Could you check a few things on this model? Use its own coordinates, in mm. A direction names the side the tool comes from. Give positions to 0.01 mm unless a question says otherwise; leave off trailing zeros. Loops run counter-clockwise (first coordinate to the right, second up) from the corner with the lowest first, then second, coordinate; pieces in that order, holes last. Notation, with made-up numbers: M 0,74 L 33,74 A18 ccw 33,99 Z; hole C 16.25,-30.75 d3. An arc over 180 degrees is marked long. Use CSV: the item, a comma, the result in double quotes.
```python
from build123d import *

# Parameters (mm, degrees)
PAD_DEPTH       = 4
SKETCH001_R     = 3.75
PAD001_DEPTH    = 9
SKETCH002_R     = 2.15
POCKET_DEPTH    = 7
CHAMFER_SIZE    = 1.5
CHAMFER001_SIZE = 1.5
CHAMFER002_SIZE = 1.5
FILLET_R        = 5
FILLET001_R     = 5


with BuildPart() as part:
    # Sketch → Pad (new body)
    with BuildSketch(Plane.XY):
        Polygon((0, 0), (20, 0), (30, 10), (30, 20), (20, 30), (0, 30), align=None)
        with BuildLine():
            ThreePointArc((4.5, 6.5), (3, 5), (4.5, 3.5))
            Line((4.5, 3.5), (7, 3.5))
            ThreePointArc((7, 3.5), (8.5, 5), (7, 6.5))
            Line((7, 6.5), (4.5, 6.5))
        make_face(mode=Mode.SUBTRACT)
        with BuildLine():
            ThreePointArc((4.5, 26.5), (3, 25), (4.5, 23.5))
            Line((4.5, 23.5), (7, 23.5))
            ThreePointArc((7, 23.5), (8.5, 25), (7, 26.5))
            Line((7, 26.5), (4.5, 26.5))
        make_face(mode=Mode.SUBTRACT)
        with BuildLine():
            ThreePointArc((23.5, 16.5), (22, 15), (23.5, 13.5))
            Line((23.5, 13.5), (26, 13.5))
            ThreePointArc((26, 13.5), (27.5, 15), (26, 16.5))
            Line((26, 16.5), (23.5, 16.5))
        make_face(mode=Mode.SUBTRACT)
    extrude(amount=PAD_DEPTH)

    # Sketch001 → Pad001 (join)
    with BuildSketch(Plane.XY):
        with Locations((15, 25.5)):
            Circle(SKETCH001_R)
        with Locations((15, 4.5)):
            Circle(SKETCH001_R)
    extrude(amount=PAD001_DEPTH)

    # Sketch002 → Pocket (cut)
    with BuildSketch(Plane.XY.offset(9)):
        with Locations((15, 25.5)):
            Circle(SKETCH002_R)
        with Locations((15, 4.5)):
            Circle(SKETCH002_R)
    extrude(amount=-POCKET_DEPTH, mode=Mode.SUBTRACT)

    # Chamfer
    chamfer_edges = [part.edges().sort_by_distance(p)[0] for p in [
        (3, 5, 4),
        (5.75, 6.5, 4),
        (8.5, 5, 4),
        (5.75, 3.5, 4),
    ]]
    chamfer(chamfer_edges, length=CHAMFER_SIZE)

    # Chamfer001
    chamfer001_edges = [part.edges().sort_by_distance(p)[0] for p in [
        (3, 25, 4),
        (5.75, 26.5, 4),
        (8.5, 25, 4),
        (5.75, 23.5, 4),
    ]]
    chamfer(chamfer001_edges, length=CHAMFER001_SIZE)

    # Chamfer002
    chamfer002_edges = [part.edges().sort_by_distance(p)[0] for p in [
        (22, 15, 4),
        (24.75, 16.5, 4),
        (27.5, 15, 4),
        (24.75, 13.5, 4),
    ]]
    chamfer(chamfer002_edges, length=CHAMFER002_SIZE)

    # Fillet
    fillet_edges = [part.edges().sort_by_distance(p)[0] for p in [
        (0, 0, 2),
        (20, 0, 2),
        (30, 10, 2),
    ]]
    fillet(fillet_edges, radius=FILLET_R)

    # Fillet001
    fillet001_edges = [part.edges().sort_by_distance(p)[0] for p in [
        (30, 20, 2),
        (20, 30, 2),
        (0, 30, 2),
    ]]
    fillet(fillet001_edges, radius=FILLET001_R)


solid = part.part
```
1. I want a section at A-A, the plane x = 6. List the corners of the cut face in (y, z) for me, then the cut area to 3 significant figures.
Outcome:
outline,"M 0,0 L 3.5,0 L 3.5,2.5 L 2,4 L 0,4 Z; M 6.5,0 L 23.5,0 L 23.5,2.5 L 22,4 L 8,4 L 6.5,2.5 Z; M 26.5,0 L 30,0 L 30,4 L 28,4 L 26.5,2.5 Z"
area,"91.5 mm2"
2. I want a section at C-C, the plane y = 15. List the corners of the cut face in (x, z) for me, then the cut area to 4 significant figures.
Outcome:
outline,"M 0,0 L 22,0 L 22,2.5 L 20.5,4 L 0,4 Z; M 27.5,0 L 30,0 L 30,4 L 29,4 L 27.5,2.5 Z"
area,"95.75 mm2"
3. Which directions (+Z, -Z, +X, -X, +Y, -Y) give clear straight access to the entire face, cutting with the end or side of a thin tool? Please do faces 1 (the face through (3, 25, 1)), 2 (the face through (1, 28, 2)), 3 (the face through (6, 3, 3)).
Outcome:
face 1,"+Z, -Z"
face 2,"+Z, -Z, -X, +Y"
face 3,"+Z"
4. I want a section at D-D, the plane z = 7.25. List the corners of the cut face in (x, y) for me.
Outcome:
outline,"C 15,4.5 d7.5; C 15,25.5 d7.5; hole C 15,4.5 d4.3; hole C 15,25.5 d4.3"
5. I'm going to push flat-ended pins straight in: pin 1 Ø5 at (x, y) = (15, 4.5) entering from +Z; pin 2 Ø1 at (x, y) = (7.5, 26) entering from +Z; pin 3 Ø2.5 at (x, y) = (15, 25.5) entering from +Z; pin 4 Ø0.8 at (x, z) = (25.5, 1) entering from -Y. Where does each tip first touch, or does it pass through?
Outcome:
pin 1,"z = 9"
pin 2,"z = 2.62"
pin 3,"z = 2"
pin 4,"y = 5.1"
6. I want a section at B-B, the plane z = 3.5. List the corners of the cut face in (x, y) for me.
Outcome:
outline,"M 0,5 A5 ccw 5,0 L 17.93,0 A5 ccw 21.46,1.46 L 28.54,8.54 A5 ccw 30,12.07 L 30,17.93 A5 ccw 28.54,21.46 L 21.46,28.54 A5 ccw 17.93,30 L 5,30 A5 ccw 0,25 Z; hole M 4.5,2.5 L 7,2.5 A2.5 ccw 7,7.5 L 4.5,7.5 A2.5 ccw Z; hole M 4.5,22.5 L 7,22.5 A2.5 ccw 7,27.5 L 4.5,27.5 A2.5 ccw Z; hole C 15,4.5 d4.3; hole C 15,25.5 d4.3; hole M 23.5,12.5 L 26,12.5 A2.5 ccw 26,17.5 L 23.5,17.5 A2.5 ccw Z"
7. Please list where these lines run through material, in increasing order: line 1 (Y direction, x = 15, z = 7.5); line 2 (Y direction, x = 15, z = 3.5); line 3 (X direction, y = 24.75, z = 3).
Outcome:
line 1,"0.75 to 2.35, 6.65 to 8.25, 21.75 to 23.35, 27.65 to 29.25"
line 2,"0 to 2.35, 6.65 to 23.35, 27.65 to 30"
line 3,"0 to 2.52, 8.98 to 12.99, 17.01 to 25.25"
8. If we mould it in two halves opening along Y, with no side actions, what happens to faces 4 (the face through (3, 5, 1)), 5 (the face through (15, 15, 0)), 6 (the face through (12, 30, 2))? For each: +Y half, -Y half, draft (parallel to the pull), parting line (faces both ways), or undercut.
Outcome:
face 4,"undercut"
face 5,"draft"
face 6,"+Y half"
